Model file for the job. Use its own axes, mm. A direction names the side the tool comes from. Give positions to 0.01 mm unless a question says otherwise; leave off trailing zeros. Loops run counter-clockwise (first coordinate to the right, second up) from the corner with the lowest first, then second, coordinate; pieces in that order, holes last. Notation, with made-up numbers: M -4.5,81 L 46.5,81 A23 ccw 46.5,99 Z; hole C -31,48.25 d8. An arc over 180 degrees is marked long. Use CSV: the item, a comma, the result in double quotes. Start each with the question number.
(1) Tool access for faces 5 (the face through (0, 9, 4.2)), 6 (the face through (-8, 9, 3)), 7 (the face through (8, 9, 3)): list every direction of +Z, -Z, +X, -X, +Y, -Y with a clear straight run to the whole face (end or side of a thin tool).
(2) Flat gauge pins, fed straight in: P1, Ø2.5, axis at x = 7, y = 4.5, coming from the -Z side; P2, Ø1.5, axis at x = -0.5, y = 11, coming from the -Z side. Where does each tip first touch, or does it go through?
(3) Wall check: line 1 along Y through (x, z) = (-7, 2.85); line 2 along X through (y, z) = (6, 4); line 3 along X through (y, z) = (6, 0.5). Give the ranges that are in metal, low to high. Write a range as from..to.
(4) Slice it at C-C on x = -6.5. List the corners of the cut face in (y, z).
(5) Two-plate mould, pull along X, no slides. Class faces 1 (the face through (3.448, 10.479, 2.028)), 2 (the face through (0, 0, 4)), 3 (the face through (-5.22, 11.96, 2.96)), 4 (the face through (-0.1, 3.5, 3.6)): pulls with the +X half, pulls with the -X half, needs draft (parallel to the pull), parting line crosses it, or undercut.
(6) Slice it at B-B on y = 4.25. State how many separate pieces and enclosed holes the cut face has, and give its area (3 significant figures).
(7) Slice it at A-A on z = 1.25. List the corners of the cut face in (x, y).
(8) Slice it at D-D on y = 11.25. List the corners of the cut face in (x, z).
```python
from build123d import *

# Parameters (mm, degrees)
SKETCH_1_W           = 22
SKETCH_1_H           = 12
EXTRUDE_1_DEPTH      = 9
FILLET_1_R           = 2
SKETCH_2_R           = 3.6
CUT_EXTRUDE_1_DEPTH  = 8
SKETCH_3_R           = 5
CUT_EXTRUDE_2_DEPTH  = 1
EXTRUDE_2_DEPTH      = 6
CUT_EXTRUDE_5_DEPTH  = 3
SKETCH_8_R           = 2.5
CUT_EXTRUDE_6_DEPTH  = 6
SKETCH_11_R          = 2
CUT_EXTRUDE_9_DEPTH  = 13
SKETCH_12_W          = 27.17111841
SKETCH_12_H          = 33.234136994
CUT_EXTRUDE_10_DEPTH = 10


with BuildPart() as part:
    # Эскиз1 → Бобышка-Вытянуть1 (new body)
    with BuildSketch(Plane(origin=(0, 0, 0), x_dir=(1, 0, 0), z_dir=(0, 1, 0))):
        Rectangle(SKETCH_1_W, SKETCH_1_H)
    extrude(amount=EXTRUDE_1_DEPTH)

    # Скругление1
    fillet_1_edges = [part.edges().sort_by_distance(p)[0] for p in [
        (11, 4.5, 6),
        (-11, 4.5, 6),
        (-11, 4.5, -6),
        (11, 4.5, -6),
    ]]
    fillet(fillet_1_edges, radius=FILLET_1_R)

    # Эскиз2 → Вырез-Вытянуть1 (cut)
    with BuildSketch(Plane(origin=(0, 0, 0), x_dir=(1, 0, 0), z_dir=(0, 1, 0))):
        Circle(SKETCH_2_R)
    extrude(amount=CUT_EXTRUDE_1_DEPTH, mode=Mode.SUBTRACT)

    # Эскиз3 → Вырез-Вытянуть2 (cut, symmetric)
    with BuildSketch(Plane.XZ.offset(-8)):
        Circle(SKETCH_3_R)
    extrude(amount=CUT_EXTRUDE_2_DEPTH, both=True, mode=Mode.SUBTRACT)

    # Эскиз6 → Бобышка-Вытянуть2 (add)
    with BuildSketch(Plane(origin=(0, 9, 0), x_dir=(1, 0, 0), z_dir=(0, 1, 0))):
        Polygon((6.92820323, 0), (3.464101615, 6), (-3.464101615, 6), (-6.92820323, 0), (-3.464101615, -6), (3.464101615, -6), align=None)
    extrude(amount=EXTRUDE_2_DEPTH)

    # Эскиз7 → Вырез-Вытянуть5 (cut)
    with BuildSketch(Plane(origin=(0, 9, 0), x_dir=(1, 0, 0), z_dir=(0, 1, 0))):
        Polygon((4.618802154, 0), (2.309401077, 4), (-2.309401077, 4), (-4.618802154, 0), (-2.309401077, -4), (2.309401077, -4), align=None)
    extrude(amount=CUT_EXTRUDE_5_DEPTH, mode=Mode.SUBTRACT)

    # Эскиз8 → Вырез-Вытянуть6 (cut)
    with BuildSketch(Plane(origin=(0, 9, 0), x_dir=(1, 0, 0), z_dir=(0, 1, 0))):
        Circle(SKETCH_8_R)
    extrude(amount=CUT_EXTRUDE_6_DEPTH, mode=Mode.SUBTRACT)

    # Эскиз11 → Вырез-Вытянуть9 (cut, through all)
    with BuildSketch(Plane(origin=(0, 0, -6), x_dir=(-1, 0, 0), z_dir=(0, 0, -1))):
        with Locations((7, 4.5)):
            Circle(SKETCH_11_R)
    cut_extrude_9 = extrude(amount=-CUT_EXTRUDE_9_DEPTH, mode=Mode.SUBTRACT)

    # Зеркальное отражение6: Вырез-Вытянуть9 across plane
    add(cut_extrude_9.mirror(Plane(origin=(0, 0, 0), x_dir=(0, 0, 1), z_dir=(1, 0, 0))), mode=Mode.SUBTRACT)

    # Эскиз12 → Вырез-Вытянуть10 (cut)
    with BuildSketch(Plane.XY):
        Rectangle(SKETCH_12_W, SKETCH_12_H)
    extrude(amount=-CUT_EXTRUDE_10_DEPTH, mode=Mode.SUBTRACT)


solid = part.part
```
Reply:
1,face 5,"-Z"
1,face 6,"+Z, -X, +Y"
1,face 7,"+Z, +X, +Y"
2,P1,"passes through"
2,P2,"stops at z = 4"
3,line 1,"y = 0..2.5, 6.5..9"
3,line 2,"x = -11..-8.32, -5.68..5.68, 8.32..11"
3,line 3,"x = -11..-8.32, -5.68..-3.57, 3.57..5.68, 8.32..11"
4,outline,"M 0,0 L 2.56,0 L 2.56,6 L 0,6 Z; M 6.44,0 L 15,0 L 15,0.74 L 9,0.74 L 9,6 L 6.44,6 Z"
5,face 1,"undercut"
5,face 2,"needs draft"
5,face 3,"pulls with the -X half"
5,face 4,"undercut"
6,separate pieces,"3"
6,enclosed holes,"0"
6,area,"62.3 mm^2"
7,outline,"M -11,0 L -3.38,0 L -3.38,7 L -4.84,7 L -4.84,9 L -3.9,9 L -3.9,12 L -2.17,12 L -2.17,15 L -6.21,15 L -6.21,9 L -11,9 Z; M 2.17,12 L 3.9,12 L 3.9,9 L 4.84,9 L 4.84,7 L 3.38,7 L 3.38,0 L 11,0 L 11,9 L 6.21,9 L 6.21,15 L 2.17,15 Z; hole C -7,4.5 d4; hole C 7,4.5 d4"
8,outline,"M -6.93,0 L -4.62,0 L -2.31,4 L 2.31,4 L 4.62,0 L 6.93,0 L 3.46,6 L -3.46,6 Z"
